from build123d import *

# Parameters (mm, degrees)
BOSS_EXTRUDE1_DEPTH = 12
SKETCH2_R           = 37.5
CUT_EXTRUDE1_DEPTH  = 22
SKETCH5_R           = 7
CUT_EXTRUDE3_DEPTH  = 22
SKETCH6_R           = 70
BOSS_EXTRUDE2_DEPTH = 65
CUT_EXTRUDE4_START  = -80
SKETCH7_R           = 37.5
CUT_EXTRUDE4_DEPTH  = 80
SKETCH9_R           = 55
CUT_EXTRUDE5_DEPTH  = 72


with BuildPart() as part:
    # Sketch1 → Boss-Extrude1 (new body)
    with BuildSketch(Plane(origin=(0, 0, 0), x_dir=(1, 0, 0), z_dir=(0, 1, 0))):
        with BuildLine():
            Line((66.645984298, 85.104941493), (128.643951995, -22.278688525))
            ThreePointArc((128.643951995, -22.278688525), (128.643951995, -62.278688525), (94.002935844, -82.278688525))
            Line((94.002935844, -82.278688525), (-29.992999551, -82.278688525))
            ThreePointArc((-29.992999551, -82.278688525), (-64.634015702, -62.278688525), (-64.634015702, -22.278688525))
            Line((-64.634015702, -22.278688525), (-2.636048005, 85.104941493))
            ThreePointArc((-2.636048005, 85.104941493), (32.004968146, 105.104941493), (66.645984298, 85.104941493))
        make_face()
    extrude(amount=BOSS_EXTRUDE1_DEPTH)

    # Sketch2 → Cut-Extrude1 (cut)
    with BuildSketch(Plane(origin=(0, 12, 0), x_dir=(1, 0, 0), z_dir=(0, 1, 0))):
        with Locations(Location((32.004968146, -4.752094378, 0), (0, 0, 270))):
            Circle(SKETCH2_R)
    extrude(amount=-CUT_EXTRUDE1_DEPTH, mode=Mode.SUBTRACT)

    # Sketch5 → Cut-Extrude3 (cut)
    with BuildSketch(Plane(origin=(0, 12, 0), x_dir=(1, 0, 0), z_dir=(0, 1, 0))):
        with Locations(Location((109.504968146, -49.49674024, 0), (0, 0, 270))):
            Circle(SKETCH5_R)
        with Locations(Location((32.004968146, 84.737197347, 0), (0, 0, 270))):
            Circle(SKETCH5_R)
        with Locations(Location((-45.495031854, -49.49674024, 0), (0, 0, 270))):
            Circle(SKETCH5_R)
    extrude(amount=-CUT_EXTRUDE3_DEPTH, mode=Mode.SUBTRACT)

    # Sketch6 → Boss-Extrude2 (add)
    with BuildSketch(Plane(origin=(0, 12, 0), x_dir=(1, 0, 0), z_dir=(0, 1, 0))):
        with Locations(Location((32.004968146, -4.752094378, 0), (0, 0, 270))):
            Circle(SKETCH6_R)
    extrude(amount=BOSS_EXTRUDE2_DEPTH)

    # Sketch7 → Cut-Extrude4 (cut)
    with BuildSketch(Plane(origin=(0, 12, 0), x_dir=(-1, 0, 0), z_dir=(0, -1, 0)).offset(CUT_EXTRUDE4_START)):
        with Locations(Location((-32.004968146, -4.752094378, 0), (0, 0, 270))):
            Circle(SKETCH7_R)
    extrude(amount=CUT_EXTRUDE4_DEPTH, mode=Mode.SUBTRACT)

    # Sketch9 → Cut-Extrude5 (cut)
    with BuildSketch(Plane(origin=(0, 0, 0), x_dir=(-1, 0, 0), z_dir=(0, -1, 0))):
        with Locations(Location((-32.004968146, -4.752094378, 0), (0, 0, 90))):
            Circle(SKETCH9_R)
    extrude(amount=-CUT_EXTRUDE5_DEPTH, mode=Mode.SUBTRACT)


solid = part.part
Verification items for the finished model (mm, model axes). A direction names the side the tool comes from. Give positions to 0.01 mm unless a question says otherwise; leave off trailing zeros. Write each loop counter-clockwise with the first axis right and the second up, starting at its lowest first coordinate (ties: lowest second). Pieces come first, ordered by that corner, then holes. Notation, with made-up numbers: M 24,21 L 75,21 A18 cw 75,42 Z; hole C 19.5,57.5 d1. An arc over 180 degrees is marked long. Use CSV: the item, a comma, the result in double quotes.
1) Cross-section at A-A (z = -4). Enter the section's corners in (x, y), plus the area to 3 significant figures.
Final values:
outline,"M -49.46,0 L -22.29,0 L -22.29,72 L -4.46,72 L -4.46,77 L -37.45,77 L -37.45,12 L -49.46,12 Z; M 68.47,72 L 86.3,72 L 86.3,0 L 113.47,0 L 113.47,12 L 101.46,12 L 101.46,77 L 68.47,77 Z"
area,"2,800 mm²"
2) Go/stop test with flat-tipped pins: pin 1 Ø12.5 at (x, z) = (32, -84.74) entering from +Y; pin 2 Ø16 at (x, z) = (-45.5, 49.5) entering from +Y; pin 3 Ø12 at (y, z) = (64.5, -21.5) entering from +X; pin 4 Ø10 at (y, z) = (39, 53) entering from +X. Record where each tip stops, or that it passes through.
Final values:
pin 1,"through"
pin 2,"y = 12"
pin 3,"x = 99.01"
pin 4,"x = 87.05"
3) Cross-section at B-B (y = 9). Enter the section's corners in (x, z), plus the area to 3 significant figures.
Final values:
outline,"M -64.63,22.28 L -2.64,-85.1 A40 ccw 66.65,-85.1 L 128.64,22.28 A40 ccw 94,82.28 L -29.99,82.28 A40 ccw Z; hole C -45.5,49.5 d14; hole C 32,4.75 d110; hole C 32,-84.74 d14; hole C 109.5,49.5 d14"
area,"16,600 mm²"
4) Material ranges on line 1 along Y through (x, z) = (-27, 51); line 2 along Y through (x, z) = (6, -23.5); line 3 along Z through (x, y) = (54, 11), recorded low to high.
Final values:
line 1,"0 to 12"
line 2,"72 to 77"
line 3,"-98.51 to -45.66, 55.16 to 82.28"
5) Cross-section at C-C (z = -55). Enter the section's corners in (x, y).
Final values:
outline,"M -20.02,0 L 84.03,0 L 84.03,12 L 68.47,12 L 68.47,77 L -4.46,77 L -4.46,12 L -20.02,12 Z"
6) Release check for a two-part mould opening along X. For faces 4 (the face through (105.25, 6.08, 43.94)), 5 (the face through (10.94, 35.496, -46.054)), 6 (the face through (31.4, 5.9, -105.1)), 7 (the face through (33, 6, 82.279)) record: released by +X, released by -X, zero draft, split by the parting line, or undercut.
Final values:
face 4,"undercut"
face 5,"undercut"
face 6,"split by the parting line"
face 7,"zero draft"
7) Cross-section at D-D (y = 68). Enter the section's corners in (x, z), plus the area to 3 significant figures.
Final values:
outline,"C 32,4.75 d140; hole C 32,4.75 d110"
area,"5,890 mm²"
8) Access from +Z, -Z, +X, -X, +Y, -Y to the whole of each face (thin tool, end or side, straight path). Record for faces 1 (the face through (55.1, 12, 71.4)), 2 (the face through (2, 77, 35)), 3 (the face through (-4, 72, -7)).
Final values:
face 1,"+Y"
face 2,"+Z, -Z, +X, -X, +Y"
face 3,"-Y"
